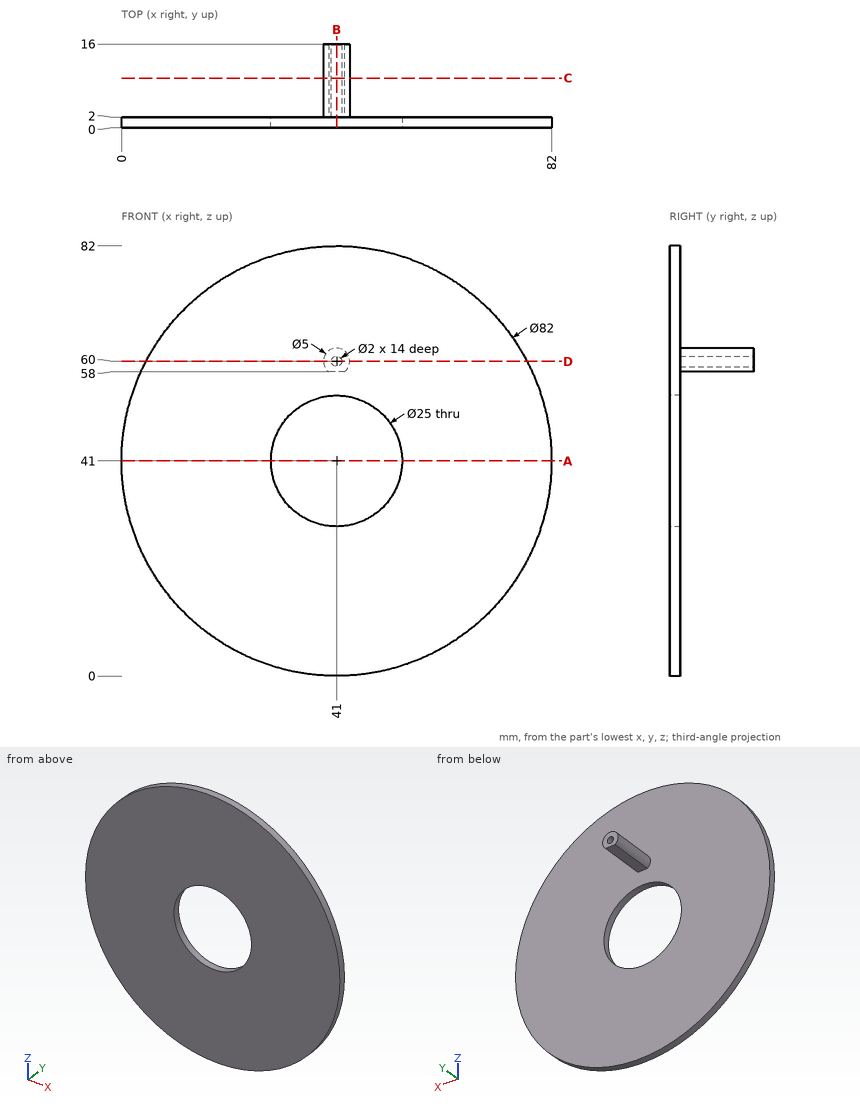
Check sheet for the drawn part. Datum: minimum x, y, z corner. Units: mm. Give positions to 0.01 mm unless a question says otherwise; leave off trailing zeros. Loops run counter-clockwise (first coordinate to the right, second up) from the corner with the lowest first, then second, coordinate; pieces in that order, holes last. Notation, with made-up numbers: (-9, 42.5) - (17, 42.5) arc R27 cw to (17, 66.5) - close; hole circle Ø1 at (62.25, 81). An arc over 180 degrees is marked (long way). Write each question's results on one line, items separated by ' | '.
1) Depth check by flat-ended pin: P1, Ø1.6, axis at x = 41, z = 60, coming from the +Y side; P2, Ø3, axis at x = 38.5, y = 10, coming from the +Z side; P3, Ø1.5, axis at y = 2.5, z = 9, coming from the +X side. Enter the tip coordinate at first touch or a pass-through.
Solution:
P1: y = 2 | P2: z = 62.29 | P3: x = 67.31
2) Sectioned sample at D-D on z = 60. Record the boundary of the cut face in (x, y).
Solution:
outline: (4.67, 0) - (77.33, 0) - (77.33, 2) - (43.5, 2) - (43.5, 16) - (42, 16) - (42, 2) - (40, 2) - (40, 16) - (38.5, 16) - (38.5, 2) - (4.67, 2) - close
3) Sectioned sample at B-B on x = 41. Record the boundary of the cut face in (y, z), plus the area to 3 significant figures.
Solution:
outline: (0, 0) - (2, 0) - (2, 28.5) - (0, 28.5) - close; (0, 53.5) - (2, 53.5) - (2, 58) - (16, 58) - (16, 59) - (2, 59) - (2, 61) - (16, 61) - (16, 62.5) - (2, 62.5) - (2, 82) - (0, 82) - close | area: 149 mm2
4) Material ranges on L1, parallel to Z at x = 41, y = 1.4; L2, parallel to Z at x = 41, y = 9; L3, parallel to Y at x = 78, z = 43, recorded low to high. Write a range as from..to.
Solution:
L1: 0..28.5, 53.5..82 | L2: 58..59, 61..62.5 | L3: 0..2
5) Sectioned sample at C-C on y = 9.5. Record the boundary of the cut face in (x, z).
Solution:
outline: (39.5, 58) - (42.5, 58) arc R2.5 ccw (long way) to start; hole circle Ø2 at (41, 60)
6) Sectioned sample at A-A on z = 41. Record the boundary of the cut face in (x, y).
Solution:
outline: (0, 0) - (28.5, 0) - (28.5, 2) - (0, 2) - close; (53.5, 0) - (82, 0) - (82, 2) - (53.5, 2) - close
